from build123d import *

# Parameters (mm, degrees)
SKETCH_1_R          = 23
EXTRUDE_1_DEPTH     = 23
CHAMFER_1_SIZE      = 2
CHAMFER_1_SIZE2     = 5.494954839
SKETCH_2_R          = 3.5
CUT_EXTRUDE_1_DEPTH = 40.837168574
SKETCH_2_3_R        = 5
SKETCH_2_3_R_2      = 3.5
EXTRUDE_2_DEPTH     = 32
CUT_EXTRUDE_START   = -19
SKETCH_4_R          = 21
SKETCH_4_R_2        = 5
CUT_EXTRUDE_2_DEPTH = 19
M3X0_51_D           = 2.5
M3X0_52_D           = 2.5
M3X0_52_DEPTH       = 7.5
M3X0_52_TIP         = 0.751075774
M3X0_53_D           = 2.5
SKETCH_12_R         = 4.3
CUT_EXTRUDE_3_DEPTH = 25


with BuildPart() as part:
    # Sketch 1 → Extrude 1 (new body)
    with BuildSketch(Plane(origin=(0, 0, 0), x_dir=(1, 0, 0), z_dir=(0, 1, 0))):
        with Locations(Location((0, 0, 0), (0, 0, 270))):
            Circle(SKETCH_1_R)
    extrude(amount=EXTRUDE_1_DEPTH)

    # Chamfer 1
    chamfer_1_edges = [part.edges().sort_by_distance(p)[0] for p in [
        (0, 23, -23),
    ]]
    chamfer_1_side = [part.faces().sort_by_distance(p)[0] for p in [
        (0, 11.5, -23),
    ]]
    chamfer(chamfer_1_edges, length=CHAMFER_1_SIZE, length2=CHAMFER_1_SIZE2, reference=chamfer_1_side[0])

    # Sketch 2 → Cut-Extrude 1 (cut, through all)
    with BuildSketch(Plane(origin=(0, 23, 0), x_dir=(1, 0, 0), z_dir=(0, 1, 0))):
        with Locations(Location((0, 0, 0), (0, 0, 270))):
            Circle(SKETCH_2_R)
    extrude(amount=-CUT_EXTRUDE_1_DEPTH, mode=Mode.SUBTRACT)

    # Sketch 2_3 → Extrude 2 (add)
    with BuildSketch(Plane(origin=(0, 23, 0), x_dir=(1, 0, 0), z_dir=(0, 1, 0))):
        with Locations(Location((0, 0, 0), (0, 0, 270))):
            Circle(SKETCH_2_3_R)
        with Locations(Location((0, 0, 0), (0, 0, 270))):
            Circle(SKETCH_2_3_R_2, mode=Mode.SUBTRACT)
    extrude(amount=-EXTRUDE_2_DEPTH)

    # Sketch 4 → Cut-Extrude 2 (cut)
    with BuildSketch(Plane.XZ.offset(CUT_EXTRUDE_START)):
        with Locations(Location((0, 0, 0), (0, 0, 270))):
            Circle(SKETCH_4_R)
        with Locations(Location((0, 0, 0), (0, 0, 90))):
            Circle(SKETCH_4_R_2, mode=Mode.SUBTRACT)
    extrude(amount=CUT_EXTRUDE_2_DEPTH, mode=Mode.SUBTRACT)

    # M3x0.51 (through all)
    with Locations(Plane(origin=(0, 23, 0), x_dir=(1, 0, 0), z_dir=(0, 1, 0))):
        with Locations((0, 12.5), (12.5, 0), (0, -12.5), (-12.5, 0)):
            Hole(M3X0_51_D / 2)

    # M3x0.52
    with Locations(Plane(origin=(0, 23, 0), x_dir=(1, 0, 0), z_dir=(0, 1, 0))):
        with Locations((6.062159206, 0.332038968), (0, 6), (-6, 0), (0, -6)):
            Hole(M3X0_52_D / 2, depth=M3X0_52_DEPTH)
            with Locations((0, 0, -(M3X0_52_DEPTH + M3X0_52_TIP / 2))):  # 118° drill point
                Cone(0, M3X0_52_D / 2, M3X0_52_TIP, mode=Mode.SUBTRACT)

    # M3x0.53 (through all)
    with Locations(Plane(origin=(0, 23, 0), x_dir=(1, 0, 0), z_dir=(0, 1, 0))):
        with Locations((-6.717514421, 6.717514421), (6.717514421, 6.717514421), (6.717514421, -6.717514421), (-6.717514421, -6.717514421)):
            Hole(M3X0_53_D / 2)

    # Sketch 12 → Cut-Extrude 3 (cut)
    with BuildSketch(Plane(origin=(0, 23, 0), x_dir=(1, 0, 0), z_dir=(0, 1, 0))):
        with Locations(Location((0, 0, 0), (0, 0, 270))):
            Circle(SKETCH_12_R)
    extrude(amount=-CUT_EXTRUDE_3_DEPTH, mode=Mode.SUBTRACT)


solid = part.part
Read the model definition and answer for the solid it produces. Units are mm, in the model's axes. A direction names the side the tool comes from. Coordinates: 2 decimals unless noted, no trailing zeros. Write each loop counter-clockwise with the first axis right and the second up, starting at its lowest first coordinate (ties: lowest second). Pieces come first, ordered by that corner, then holes. Notation, with made-up numbers: (49.25, 37.25) -> (96.25, 37.25) arc R25 ccw to (96.25, 73.25) -> close; hole circle Ø11 at (48, -14). An arc over 180 degrees is marked (long way). Return JSON: item names as keys, results as strings.
(1) The part is cut by section C-C on y = -6. Give the vertices of the cut face in (x, z), then the cut area to 3 significant figures.
Answers below:
{"outline": "circle Ø10 at (0, 0); hole circle Ø7 at (0, 0)", "area": "40.1 mm^2"}
(2) For a pull along X with two mould halves and no side action, classify faces 4 (the cylindrical face through (19.394, 10.353, 12.365)), 5 (the flat face through (-4, 23, 4)), 6 (the cylindrical face through (7.639, 20.972, 5.873)) as pulls with the +X half, pulls with the -X half, needs draft (parallel to the pull), parting line crosses it, or undercut.
Answers below:
{"face 4": "parting line crosses it", "face 5": "needs draft", "face 6": "undercut"}
(3) The part is cut by section A-A on y = 11.5. Give the vertices of the cut face in (x, z), then the cut area to 3 significant figures.
Answers below:
{"outline": "circle Ø46 at (0, 0); circle Ø10 at (0, 0); hole circle Ø42 at (0, 0); hole circle Ø8.6 at (0, 0)", "area": "297 mm^2"}
(4) The part is cut by section B-B on x = 0. State how many separate pieces and enclosed holes the cut face has, then the cut area to 3 significant figures.
Answers below:
{"separate pieces": "6", "enclosed holes": "0", "area": "223 mm^2"}
(5) Which of the six approach directions +Z, -Z, +X, -X, +Y, -Y give full straight-line access (tool end or side, diameter ignored) to faces 1 (the cylindrical face through (0.27, 20.03, -4.78)), 2 (the cylindrical face through (6.31, 9.63, -20.03)), 3 (the cylindrical face through (13.75, 20.97, -0.05))?
Answers below:
{"face 1": "+Y", "face 2": "-Y", "face 3": "+Y, -Y"}
(6) Consider line 1 along Z through (x, y) = (15.5, 14); line 2 along Z through (x, y) = (6, 15.5); line 3 along Z through (x, y) = (-6, 20). Determine where each line is inside the solid, lowest interval first. Write a range as from..to.
Answers below:
{"line 1": "-16.99..-14.17, 14.17..16.99", "line 2": "-22.2..-20.12, 20.12..22.2", "line 3": "-22.2..-7.74, -5.69..-1.25, 1.25..5.69, 7.74..22.2"}
(7) Each of these flat-tipped pins is pushed along its axis until it touches: P1, Ø4, axis at x = 0, z = 0, coming from the +Y side; P2, Ø5, axis at x = -7.5, z = 17.5, coming from the -Y side; P3, Ø3, axis at x = 6.72, z = 6.72, coming from the -Y side; P4, Ø2, axis at x = -8, y = 17.5, coming from the -Z side. Where does it stop, or does it pass through?
Answers below:
{"P1": "through", "P2": "y = 0", "P3": "y = 19", "P4": "z = -21.91"}
